Can you work these out from the drawing? Everything is in mm from the part's minimum corner. A direction names the side the tool comes from. Round coordinates to 2 decimals unless told otherwise and drop trailing zeros. Write each loop counter-clockwise with the first axis right and the second up, starting at its lowest first coordinate (ties: lowest second). Pieces come first, ordered by that corner, then holes. Notation, with made-up numbers: (85.5, 19.25) -> (107.5, 19.25) arc R22 cw to (107.5, 47.25) -> close; hole circle Ø4 at (17.5, 87). An arc over 180 degrees is marked (long way). Answer as CSV lines item,"result".
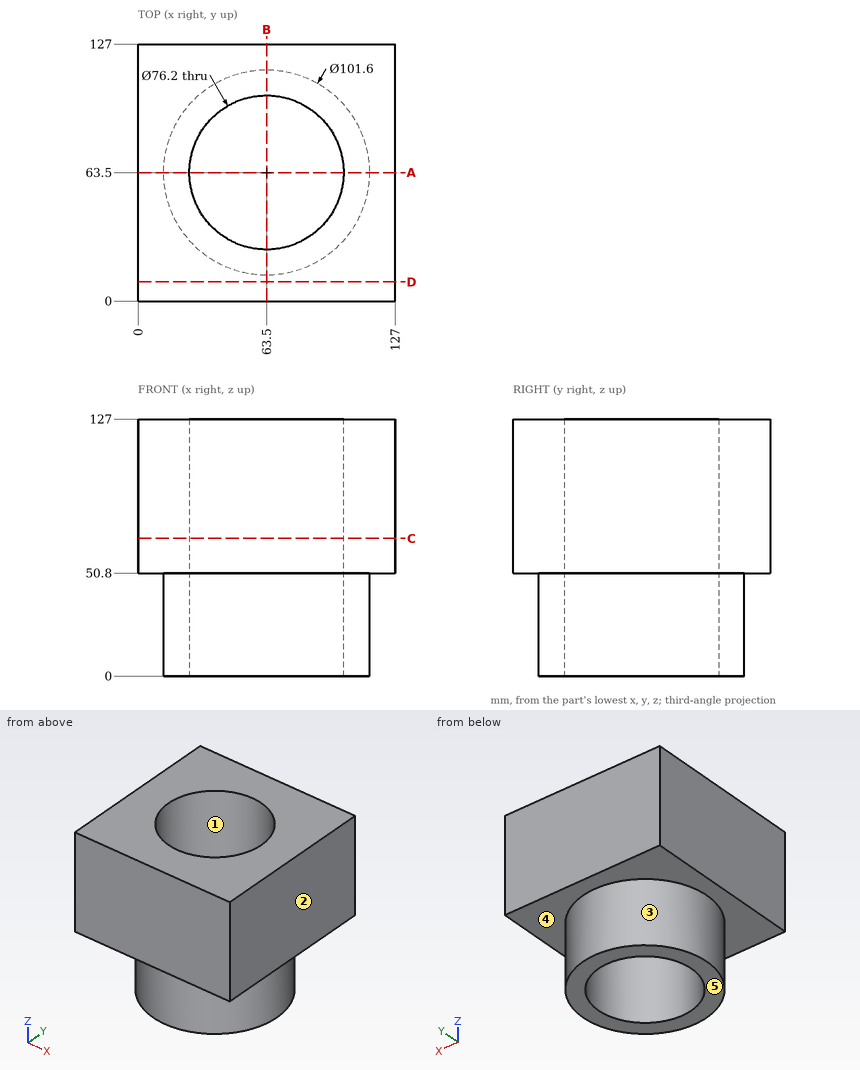
Item 1: Suppose I cut it at D-D, the plane y = 9.5. List the corners of the cut face in (x, z) for me, then the cut area to 3 significant figures.
Results found:
outline,"(0, 50.8) -> (127, 50.8) -> (127, 127) -> (0, 127) -> close"
area,"9,680 mm²"
Item 2: For the marked faces 4 and 5, which set-ups out of +Z, -Z, +X, -X, +Y, -Y let a thin tool reach every point of the face, with its end or its side?
Results found:
face 4,"-Z"
face 5,"-Z, +X, -X, +Y, -Y"
Item 3: Suppose I cut it at C-C, the plane z = 68. List the corners of the cut face in (x, y) for me.
Results found:
outline,"(0, 0) -> (127, 0) -> (127, 127) -> (0, 127) -> close; hole circle Ø76.2 at (63.5, 63.5)"
Item 4: Suppose I cut it at A-A, the plane y = 63.5. List the corners of the cut face in (x, z) for me.
Results found:
outline,"(0, 50.8) -> (12.7, 50.8) -> (12.7, 0) -> (25.4, 0) -> (25.4, 127) -> (0, 127) -> close; (101.6, 0) -> (114.3, 0) -> (114.3, 50.8) -> (127, 50.8) -> (127, 127) -> (101.6, 127) -> close"
Item 5: Will these pins go through, and if not, where does the flat tip stop? pin 1 (6 mm diameter, centred on x = 104.5, z = 28.5, fed in from -Y); pin 2 (5 mm diameter, centred on y = 66, z = 35.5, fed in from +X).
Results found:
pin 1,"stops at y = 29.79"
pin 2,"stops at x = 114.3"
Item 6: I need wall thicknesses on L1, parallel to Y at x = 63, z = 50; L2, parallel to Y at x = 63.5, z = 51. Which ranges of each line are inside material? Lowest first, please.
Results found:
L1,"y = 12.7 to 25.4, 101.6 to 114.3"
L2,"y = 0 to 25.4, 101.6 to 127"
Item 7: If we mould it in two halves opening along Y, with no side actions, what happens to the marked faces 1, 2 and 3? For each: pulls with the +Y half, pulls with the -Y half, needs draft (parallel to the pull), parting line crosses it, or undercut.
Results found:
face 1,"undercut"
face 2,"needs draft"
face 3,"parting line crosses it"
